from build123d import *

# Parameters (mm, degrees)
SKETCH1_R           = 2.7432
BOSS_EXTRUDE1_DEPTH = 17.78
SKETCH2_R           = 3.175
SKETCH2_R_2         = 1.4732
CUT_EXTRUDE1_DEPTH  = 4.064
SKETCH4_R           = 3.175
BOSS_EXTRUDE2_DEPTH = 2.9972
SKETCH5_W           = 0.635
SKETCH5_H           = 6.318170226
BOSS_EXTRUDE3_DEPTH = 12.7
SKETCH6_W           = 6.318170226
SKETCH6_H           = 0.635
BOSS_EXTRUDE4_DEPTH = 7.62
CUT_EXTRUDE2_DEPTH  = 7.62
SKETCH8_R           = 2.1209
CUT_EXTRUDE3_DEPTH  = 10.922
CUT_EXTRUDE4_START  = -6.858
SKETCH9_R           = 0.508
CUT_EXTRUDE4_DEPTH  = 6.858
SWEEP2_PITCH        = 2.54
SWEEP2_HEIGHT       = 1.143
SWEEP2_RADIUS       = 3.175
SWEEP2_START_ANGLE  = -90
SKETCH10_W          = 0.508
SKETCH10_H          = 0.762
SWEEP3_PITCH        = 2.54
SWEEP3_HEIGHT       = 1.143
SWEEP3_RADIUS       = 3.175
SWEEP3_START_ANGLE  = 90
SKETCH17_W          = 0.508
SKETCH17_H          = 0.762
SKETCH18_R          = 0.5334
SKETCH18_R_2        = 0.4064
BOSS_EXTRUDE6_DEPTH = 46.228
INTERSECT1_DEPTH    = 4.318


# Read off the part's stored shape, not the designer's step: Intersect1
with BuildPart() as part:
    # Sketch1 → Boss-Extrude1 (new body)
    with BuildSketch(Plane(origin=(0, 0, 0), x_dir=(1, 0, 0), z_dir=(0, 1, 0))):
        with Locations(Location((0, 0, 0), (0, 0, 270))):
            Circle(SKETCH1_R)
    extrude(amount=BOSS_EXTRUDE1_DEPTH)

    # Sketch2 → Cut-Extrude1 (cut)
    with BuildSketch(Plane(origin=(0, 17.78, 0), x_dir=(1, 0, 0), z_dir=(0, 1, 0))):
        Circle(SKETCH2_R)
        with Locations(Location((0, 0, 0), (0, 0, 270))):
            Circle(SKETCH2_R_2, mode=Mode.SUBTRACT)
    extrude(amount=-CUT_EXTRUDE1_DEPTH, mode=Mode.SUBTRACT)

    # Sketch3 → Cut-Revolve1 (revolve, cut)
    with BuildSketch(Plane.XY, mode=Mode.PRIVATE) as cut_revolve1_sk:
        Polygon((1.4732, 13.716), (2.7432, 10.922), (2.7432, 13.716), align=None)
    revolve(cut_revolve1_sk.sketch.rotate(Axis((0, 13.716, 0), (0, 1, 0)), 90), axis=Axis((0, 13.716, 0), (0, 1, 0)), mode=Mode.SUBTRACT)

    # Sketch4 → Boss-Extrude2 (add)
    with BuildSketch(Plane.XZ):
        with Locations(Location((0, 0, 0), (0, 0, 270))):
            Circle(SKETCH4_R)
    extrude(amount=-BOSS_EXTRUDE2_DEPTH)

    # Sketch5 → Boss-Extrude3 (add)
    with BuildSketch(Plane(origin=(0, 2.9972, 0), x_dir=(1, 0, 0), z_dir=(0, 1, 0))):
        Rectangle(SKETCH5_W, SKETCH5_H)
    extrude(amount=BOSS_EXTRUDE3_DEPTH)

    # Sketch6 → Boss-Extrude4 (add)
    with BuildSketch(Plane(origin=(0, 2.9972, 0), x_dir=(1, 0, 0), z_dir=(0, 1, 0))):
        Rectangle(SKETCH6_W, SKETCH6_H)
    extrude(amount=BOSS_EXTRUDE4_DEPTH)

    # Sketch7 → Cut-Extrude2 (cut)
    with BuildSketch(Plane(origin=(0.3175, 0, 0), x_dir=(0, 0, -1), z_dir=(1, 0, 0))):
        Polygon((1.438579852, 15.6972), (3.159085113, 14.9352), (3.159085113, 15.6972), align=None)
        Polygon((-1.438579852, 15.6972), (-3.159085113, 15.6972), (-3.159085113, 14.9352), align=None)
    extrude(amount=-CUT_EXTRUDE2_DEPTH, mode=Mode.SUBTRACT)

    # Sketch8 → Cut-Extrude3 (cut)
    with BuildSketch(Plane.XZ):
        with Locations(Location((0, 0, 0), (0, 0, 270))):
            Circle(SKETCH8_R)
    extrude(amount=-CUT_EXTRUDE3_DEPTH, mode=Mode.SUBTRACT)

    # Sketch9 → Cut-Extrude4 (cut)
    with BuildSketch(Plane(origin=(0, 17.78, 0), x_dir=(1, 0, 0), z_dir=(0, 1, 0)).offset(CUT_EXTRUDE4_START)):
        with Locations(Location((0, 0, 0), (0, 0, 270))):
            Circle(SKETCH9_R)
    extrude(amount=CUT_EXTRUDE4_DEPTH, mode=Mode.SUBTRACT)

    # Sweep2: sweep along a helix
    with BuildLine() as sweep2_path:
        add(Helix(SWEEP2_PITCH, SWEEP2_HEIGHT, SWEEP2_RADIUS, center=(0, 0.508, 0), direction=(0, 1, 0), mode=Mode.PRIVATE).rotate(Axis((0, 0.508, 0), (0, 1, 0)), SWEEP2_START_ANGLE))
    # Sketch10 → Sweep2 (sweep)
    with BuildSketch(Plane.XY):
        with Locations((-3.429, 0.889)):
            Rectangle(SKETCH10_W, SKETCH10_H)
    sweep(path=sweep2_path.line, is_frenet=True)

    # Sweep3: sweep along a helix
    with BuildLine() as sweep3_path:
        add(Helix(SWEEP3_PITCH, SWEEP3_HEIGHT, SWEEP3_RADIUS, center=(0, 0.508, 0), direction=(0, 1, 0), mode=Mode.PRIVATE).rotate(Axis((0, 0.508, 0), (0, 1, 0)), SWEEP3_START_ANGLE))
    # Sketch17 → Sweep3 (sweep)
    with BuildSketch(Plane.XY):
        with Locations((3.429, 0.889)):
            Rectangle(SKETCH17_W, SKETCH17_H)
    sweep(path=sweep3_path.line, is_frenet=True)

    # Sketch18 → Boss-Extrude6 (add)
    with BuildSketch(Plane.XZ.offset(-10.922)):
        with Locations(Location((0, 0, 0), (0, 0, 90))):
            Circle(SKETCH18_R)
        with Locations(Location((0, 0, 0), (0, 0, 270))):
            Circle(SKETCH18_R_2, mode=Mode.SUBTRACT)
    extrude(amount=-BOSS_EXTRUDE6_DEPTH)

    # Intersect1 outline → Intersect1 (cut)
    with BuildSketch(Plane(origin=(0, 0, 0), x_dir=(1, 0, 0), z_dir=(0, 1, 0))):
        with BuildLine():
            Line((-3.175, 0), (-3.683, 0))
            add(Edge.make_bspline(
                [(-3.683, 0), (-3.683, -1.196679241), (-2.97960959, -2.164813084), (-2.276219181, -3.132946927), (-1.13810959, -3.50274115), (0, -3.872535372), (1.13810959, -3.50274115), (2.276219181, -3.132946927), (2.97960959, -2.164813084), (3.322482299, -1.692889287), (3.50274115, -1.13810959)],
                knots=[0, 0, 0, 0.1, 0.1, 0.2, 0.2, 0.3, 0.3, 0.4, 0.4, 0.45, 0.45, 0.45], degree=2, weights=[1, 0.951056516, 1, 0.951056516, 1, 0.951056516, 1, 0.951056516, 1, 0.975528258, 0.975528258]))
            Line((3.50274115, -1.13810959), (3.019604439, -0.981128957))
            ThreePointArc((3.019604439, -0.981128957), (1.992470769, -2.471980023), (0.3175, -3.159085113))
            ThreePointArc((0.3175, -3.159085113), (0, -3.175), (-0.3175, -3.159085113))
            ThreePointArc((-0.3175, -3.159085113), (-2.24506403, -2.24506403), (-3.159085113, -0.3175))
            ThreePointArc((-3.159085113, -0.3175), (-3.171018782, -0.158949311), (-3.175, 0))
        make_face()
        with BuildLine():
            ThreePointArc((-3.159085113, 0.3175), (-3.171018782, 0.158949311), (-3.175, 0))
            ThreePointArc((-3.175, 0), (-3.171018782, -0.158949311), (-3.159085113, -0.3175))
            Line((-3.159085113, -0.3175), (-3.159085113, 0.3175))
        make_face()
        with BuildLine():
            ThreePointArc((0.3175, -3.159085113), (1.992470769, -2.471980023), (3.019604439, -0.981128957))
            ThreePointArc((3.019604439, -0.981128957), (3.107113129, -0.653049008), (3.159085113, -0.3175))
            Line((3.159085113, -0.3175), (2.724764208, -0.3175))
            ThreePointArc((2.724764208, -0.3175), (1.939735322, -1.939735322), (0.3175, -2.724764208))
            Line((0.3175, -2.724764208), (0.3175, -3.159085113))
        make_face()
        with BuildLine():
            ThreePointArc((-3.019604439, 0.981128957), (-3.107113129, 0.653049008), (-3.159085113, 0.3175))
            Line((-3.159085113, 0.3175), (-2.724764208, 0.3175))
            ThreePointArc((-2.724764208, 0.3175), (-1.939735322, 1.939735322), (-0.3175, 2.724764208))
            Line((-0.3175, 2.724764208), (-0.3175, 3.159085113))
            ThreePointArc((-0.3175, 3.159085113), (-1.992470769, 2.471980023), (-3.019604439, 0.981128957))
        make_face()
        with BuildLine():
            Line((-2.724764208, 0.3175), (-3.159085113, 0.3175))
            Line((-3.159085113, 0.3175), (-3.159085113, -0.3175))
            Line((-3.159085113, -0.3175), (-2.724764208, -0.3175))
            ThreePointArc((-2.724764208, -0.3175), (-2.7432, 0), (-2.724764208, 0.3175))
        make_face()
        with BuildLine():
            Line((-2.724764208, -0.3175), (-3.159085113, -0.3175))
            ThreePointArc((-3.159085113, -0.3175), (-2.24506403, -2.24506403), (-0.3175, -3.159085113))
            Line((-0.3175, -3.159085113), (-0.3175, -2.724764208))
            ThreePointArc((-0.3175, -2.724764208), (-1.939735322, -1.939735322), (-2.724764208, -0.3175))
        make_face()
        with BuildLine():
            Line((-0.3175, -3.159085113), (0.3175, -3.159085113))
            Line((0.3175, -3.159085113), (0.3175, -2.724764208))
            Line((0.3175, -2.724764208), (0.3175, -2.097000372))
            ThreePointArc((0.3175, -2.097000372), (0, -2.1209), (-0.3175, -2.097000372))
            Line((-0.3175, -2.097000372), (-0.3175, -2.724764208))
            Line((-0.3175, -2.724764208), (-0.3175, -3.159085113))
        make_face()
        with BuildLine():
            ThreePointArc((-0.3175, -3.159085113), (0, -3.175), (0.3175, -3.159085113))
            Line((0.3175, -3.159085113), (-0.3175, -3.159085113))
        make_face()
        with BuildLine():
            Line((3.159085113, 0.3175), (3.159085113, -0.3175))
            ThreePointArc((3.159085113, -0.3175), (3.171018782, -0.158949311), (3.175, 0))
            ThreePointArc((3.175, 0), (3.171018782, 0.158949311), (3.159085113, 0.3175))
        make_face()
        with BuildLine():
            Line((2.724764208, -0.3175), (3.159085113, -0.3175))
            Line((3.159085113, -0.3175), (3.159085113, 0.3175))
            Line((3.159085113, 0.3175), (2.724764208, 0.3175))
            ThreePointArc((2.724764208, 0.3175), (2.7432, 0), (2.724764208, -0.3175))
        make_face()
        with BuildLine():
            Line((-3.50274115, 1.13810959), (-3.019604439, 0.981128957))
            ThreePointArc((-3.019604439, 0.981128957), (-1.992470769, 2.471980023), (-0.3175, 3.159085113))
            ThreePointArc((-0.3175, 3.159085113), (0, 3.175), (0.3175, 3.159085113))
            ThreePointArc((0.3175, 3.159085113), (2.24506403, 2.24506403), (3.159085113, 0.3175))
            ThreePointArc((3.159085113, 0.3175), (3.171018782, 0.158949311), (3.175, 0))
            Line((3.175, 0), (3.683, 0))
            add(Edge.make_bspline(
                [(3.683, 0), (3.683, 1.196679241), (2.97960959, 2.164813084), (2.276219181, 3.132946927), (1.13810959, 3.50274115), (0, 3.872535372), (-1.13810959, 3.50274115), (-2.276219181, 3.132946927), (-2.97960959, 2.164813084), (-3.322482299, 1.692889287), (-3.50274115, 1.13810959)],
                knots=[0, 0, 0, 0.1, 0.1, 0.2, 0.2, 0.3, 0.3, 0.4, 0.4, 0.45, 0.45, 0.45], degree=2, weights=[1, 0.951056516, 1, 0.951056516, 1, 0.951056516, 1, 0.951056516, 1, 0.975528258, 0.975528258]))
        make_face()
        with BuildLine():
            ThreePointArc((-0.3175, 2.724764208), (-1.939735322, 1.939735322), (-2.724764208, 0.3175))
            ThreePointArc((-2.724764208, 0.3175), (-2.7432, 0), (-2.724764208, -0.3175))
            ThreePointArc((-2.724764208, -0.3175), (-1.939735322, -1.939735322), (-0.3175, -2.724764208))
            Line((-0.3175, -2.724764208), (-0.3175, -2.097000372))
            ThreePointArc((-0.3175, -2.097000372), (-2.1209, 0), (-0.3175, 2.097000372))
            Line((-0.3175, 2.097000372), (-0.3175, 2.724764208))
        make_face()
        with BuildLine():
            Line((0.3175, -2.097000372), (0.3175, -2.724764208))
            ThreePointArc((0.3175, -2.724764208), (1.939735322, -1.939735322), (2.724764208, -0.3175))
            ThreePointArc((2.724764208, -0.3175), (2.7432, 0), (2.724764208, 0.3175))
            ThreePointArc((2.724764208, 0.3175), (1.939735322, 1.939735322), (0.3175, 2.724764208))
            Line((0.3175, 2.724764208), (0.3175, 2.097000372))
            ThreePointArc((0.3175, 2.097000372), (1.608042686, 1.382901128), (2.1209, 0))
            ThreePointArc((2.1209, 0), (1.608042686, -1.382901128), (0.3175, -2.097000372))
        make_face()
        with BuildLine():
            Line((2.724764208, 0.3175), (3.159085113, 0.3175))
            ThreePointArc((3.159085113, 0.3175), (2.24506403, 2.24506403), (0.3175, 3.159085113))
            Line((0.3175, 3.159085113), (0.3175, 2.724764208))
            ThreePointArc((0.3175, 2.724764208), (1.939735322, 1.939735322), (2.724764208, 0.3175))
        make_face()
        with BuildLine():
            ThreePointArc((0.3175, 3.159085113), (0, 3.175), (-0.3175, 3.159085113))
            Line((-0.3175, 3.159085113), (0.3175, 3.159085113))
        make_face()
        with BuildLine():
            Line((0.3175, 3.159085113), (-0.3175, 3.159085113))
            Line((-0.3175, 3.159085113), (-0.3175, 2.724764208))
            Line((-0.3175, 2.724764208), (-0.3175, 2.097000372))
            ThreePointArc((-0.3175, 2.097000372), (0, 2.1209), (0.3175, 2.097000372))
            Line((0.3175, 2.097000372), (0.3175, 2.724764208))
            Line((0.3175, 2.724764208), (0.3175, 3.159085113))
        make_face()
    extrude(amount=INTERSECT1_DEPTH, mode=Mode.SUBTRACT)


solid = part.part
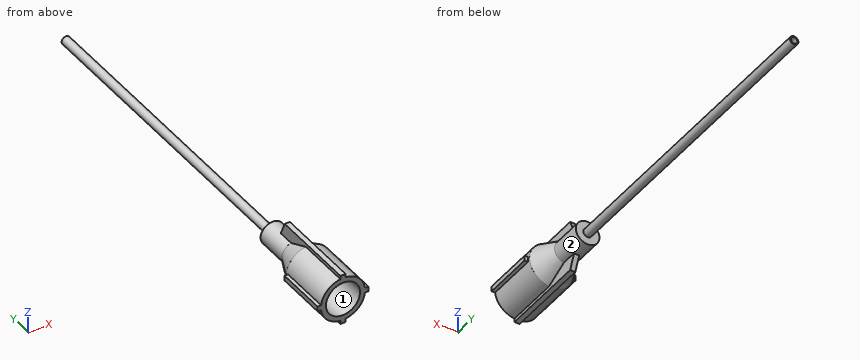
Part model, mm, in its own coordinate system. Face numbers are marked on the shaded views. Coordinates: 2 decimals unless noted, no trailing zeros. Write each loop counter-clockwise with the first axis right and the second up, starting at its lowest first coordinate (ties: lowest second). Pieces come first, ordered by that corner, then holes. Notation, with made-up numbers: M -12,22.5 L 27,22.5 A12 ccw 27,42.5 Z; hole C -22.75,4.5 d10. An arc over 180 degrees is marked long. Return JSON: item names as keys, results as strings.
1. Probe L1, parallel to X at y = 9, z = 0; L2, parallel to X at y = 7, z = 1.5. List the from-to ranges inside material, lowest first.
Determined:
{"L1": "-3.16 to -2.12, 2.12 to 3.16", "L2": "-2.3 to -1.5, 1.5 to 2.3"}
2. Pull direction Z, two halves, no side cores. Call the marked faces 1 and 2: pulls with the +Z half, pulls with the -Z half, needs draft (parallel to the pull), parting line crosses it, or undercut.
Determined:
{"face 1": "undercut", "face 2": "parting line crosses it"}
3. Saw through at A-A, the plane y = 35.5. Write the cut outline in (x, z).
Determined:
{"outline": "C 0,0 d1.07; hole C 0,0 d0.81"}
4. Flat gauge pins, fed straight in: pin 1 Ø0.5 at (y, z) = (10.5, -2) entering from +X; pin 2 Ø2 at (x, z) = (-2, 1) entering from +Y; pin 3 Ø1.5 at (y, z) = (31, -1.5) entering from -X; pin 4 Ø2 at (x, z) = (0.5, 0.5) entering from -Y. Where does each tip first touch, or does it go through?
Determined:
{"pin 1": "x = 2.11", "pin 2": "y = 17.78", "pin 3": "through", "pin 4": "y = 10.92"}
